from build123d import *

# Parameters (mm, degrees)
F0_R     = 7.5
F1_DEPTH = 8
F2_R     = 6.75
F3_DEPTH = 2
F5_DEPTH = 4
F6_R     = 3.5
F7_DEPTH = 12
F8_R     = 2.6
F9_DEPTH = 12


with BuildPart() as f1:
    # F0 (on Top) → F1 (new body)
    with BuildSketch(Plane.XY):
        Circle(F0_R)
    extrude(amount=F1_DEPTH)

    # F2 (on face) → F3 (cut)
    with BuildSketch(Plane.XY.offset(8)):
        Circle(F2_R)
    extrude(amount=-F3_DEPTH, mode=Mode.SUBTRACT)

    # F4 (on face) → F5 (cut)
    with BuildSketch(Plane.XY.offset(6)):
        Polygon((6.060904, 0.124281), (2.922821, 5.311037), (-3.138083, 5.186756), (-6.060904, -0.124281), (-2.922821, -5.311037), (3.138083, -5.186756), align=None)
    extrude(amount=-F5_DEPTH, mode=Mode.SUBTRACT)

    # F6 (on face) → F7 (join)
    with BuildSketch(Plane(origin=(0, 0, 0), x_dir=(1, 0, 0), z_dir=(0, 0, -1))):
        Circle(F6_R)
    extrude(amount=F7_DEPTH)

    # F8 (on face) → F9 (cut)
    with BuildSketch(Plane(origin=(0, 0, -12), x_dir=(1, 0, 0), z_dir=(0, 0, -1))):
        Circle(F8_R)
    extrude(amount=-F9_DEPTH, mode=Mode.SUBTRACT)


solid = f1.part
Could you check a few things on this model? Use its own coordinates, in mm. A direction names the side the tool comes from. Round coordinates to 2 decimals unless told otherwise and drop trailing zeros. Loops run counter-clockwise (first coordinate to the right, second up) from the corner with the lowest first, then second, coordinate; pieces in that order, holes last. Notation, with made-up numbers: (76.25, 4) - (127.25, 4) arc R19 ccw to (127.25, 39) - close; hole circle Ø4 at (-2, 45.5). An arc over 180 degrees is marked (long way). Write item = value, one per line.
1) Imagine slicing it at A-A (y = -4.25). Please give me the cut outline in (x, z).
Computed:
outline = (-6.18, 0) - (6.18, 0) - (6.18, 8) - (5.24, 8) - (5.24, 6) - (3.65, 6) - (3.65, 2) - (-3.56, 2) - (-3.56, 6) - (-5.24, 6) - (-5.24, 8) - (-6.18, 8) - close
2) Imagine slicing it at B-B (x = 0.5). Please give me the cut outline in (y, z).
Computed:
outline = (-7.48, 0) - (-3.46, 0) - (-3.46, -12) - (-2.55, -12) - (-2.55, 0) - (2.55, 0) - (2.55, -12) - (3.46, -12) - (3.46, 0) - (7.48, 0) - (7.48, 8) - (6.73, 8) - (6.73, 6) - (5.26, 6) - (5.26, 2) - (-5.24, 2) - (-5.24, 6) - (-6.73, 6) - (-6.73, 8) - (-7.48, 8) - close
3) I need wall thicknesses on line 1 along Y through (x, z) = (0, -2.5); line 2 along Y through (x, z) = (0, 7); line 3 along Z through (x, y) = (0.5, 1.75). Which ranges of each line are inside material? Lowest first, please. Write a range as from..to.
Computed:
line_1 = -3.5..-2.6, 2.6..3.5
line_2 = -7.5..-6.75, 6.75..7.5
line_3 = 0..2
4) On a 3-axis mill with a long thin cutter (end or side, diameter ignored), from which of +Z, -Z, +X, -X, +Y, -Y can I reach the whole of each face in a straight line? I mean faces 1 (the flat face through (-7, 1, 8)), 2 (the cylindrical face through (-0.338, -2.578, -6.084)), 3 (the flat face through (-5, 3, 6)). Say none if no direction works.
Computed:
face_1 = +Z, +X, -X, +Y, -Y
face_2 = -Z
face_3 = +Z
5) If we mould it in two halves opening along Y, with no side actions, what happens to faces 4 (the flat face through (3.2, 1.8, 0)), 5 (the cylindrical face through (-7.493, 0.33, 3.944)), 6 (the flat face through (4.58, -2.57, 4.03))? For each: pulls with the +Y half, pulls with the -Y half, needs draft (parallel to the pull), parting line crosses it, or undercut.
Computed:
face_4 = needs draft
face_5 = parting line crosses it
face_6 = undercut
6) I'm going to push flat-ended pins straight in: P1, Ø5, axis at x = 5, z = -7.5, coming from the +Y side; P2, Ø8, axis at x = -2.5, z = -8, coming from the +Y side; P3, Ø8, axis at y = 2.5, z = -0.5, coming from the -X side; P4, Ø6, axis at y = 5.5, z = -5.5, coming from the +X side. Where does each tip first touch, or does it pass through?
Computed:
P1 = 2.45
P2 = 3.5
P3 = -7.5
P4 = 2.45
7) Imagine slicing it at D-D (y = 3.25). Please give me the cut outline in (x, z).
Computed:
outline = (-6.76, 0) - (-1.3, 0) - (-1.3, -12) - (1.3, -12) - (1.3, 0) - (6.76, 0) - (6.76, 8) - (5.92, 8) - (5.92, 6) - (4.17, 6) - (4.17, 2) - (-4.2, 2) - (-4.2, 6) - (-5.92, 6) - (-5.92, 8) - (-6.76, 8) - close
8) Imagine slicing it at C-C (z = -7.5). Please give me the cut outline in (x, y), and give its area (3 significant figures).
Computed:
outline = circle Ø7 at (0, 0); hole circle Ø5.2 at (0, 0)
area = 17.2 mm2
